Autodesk Inventor part; units mm, degrees
ref_plane "Work Plane4" through (164.3995, -80, 0) normal (0, 0, 1) x (1, 0, 0)
ref_plane "YZ Plane" through (0, 0, 0) normal (1, 0, 0) x (0, 1, 0)
ref_plane "XZ Plane" through (0, 0, 0) normal (0, 1, 0) x (-1, 0, 0)
ref_plane "Work Plane4" through (164.3995, -80, 0) normal (0, 0, 1) x (1, 0, 0)
sketch "Sketch1" plane through (164.3995, -80, 0) normal (0, 0, 1) x (1, 0, 0)
  circle A0 centre (-12.7, -38.1) radius 4.5
  circle A1 centre (-12.7, -12.7) radius 4.5
  circle A2 centre (-176.0991, -12.7) radius 4.5
  circle A3 centre (-176.0991, -38.1) radius 4.5
  line L0 (0, -50.8) -> (-188.7991, -50.8)
  line L1 (0, 0) -> (0, -50.8)
  line L2 (-188.7991, 0) -> (0, 0)
  line L3 (-188.7991, 0) -> (-188.7991, -50.8)
  circle A4 centre (-94.3995, 37) radius 4.7625
  circle A5 centre (-134.3995, 37) radius 2.489
  circle A6 centre (-54.3995, 37) radius 2.489
  line L4 (-26.3995, 25) -> (-162.3995, 25)
  line L5 (-26.3995, 49) -> (-26.3995, 25)
  line L6 (-162.3995, 49) -> (-26.3995, 49)
  line L7 (-162.3995, 25) -> (-162.3995, 49)
  line L8 (-26.3995, 25) -> (0, 0)
  line L9 (-162.3995, 25) -> (-188.7991, 0)
  point P0 (-94.3995, 0)
  dimension "d5" = 136
  dimension "d6" = 24
  dimension "d7" = 28
  dimension "d8" = 12
  dimension "d9" = 12
  dimension "d10" = 68
  dimension "d11" = 40
  dimension "d12" = 12
  dimension "d13" = 25
  dimension "d14" = 9.525
  dimension "d15" = 4.978
  dimension "d16" = 4.978
extrude "Extrusion1" add sketch "Sketch1" along normal blind 10
fillet "Fillet3" radius 2 8 edges at (70, -130.8, 10) (164.3995, -105.4, 10) (151.1998, -67.5, 10) (138, -43, 10) (70, -31, 10) (2, -43, 10) (-11.1998, -67.5, 10) (-24.3995, -105.4, 10)
properties part number "1136_RU Top Plate_V1" material "Aluminum"
Design review of the part built by this model. Coordinates are the model's own, in mm. A direction names the side the tool comes from. Coordinates: 2 decimals unless noted, no trailing zeros. Loops run counter-clockwise (first coordinate to the right, second up) from the corner with the lowest first, then second, coordinate; pieces in that order, holes last.
Q1. For pin 1 (3 mm diameter, centred on x = 30, y = -43, fed in from +Z); pin 2 (3 mm diameter, centred on y = -49, z = 6, fed in from +X), all flat-tipped, find the tip position at first contact; note any pin that passes through.
Reported:
pin 1: passes through
pin 2: stops at x = 138
Q2. To check wall thickness, follow line 1 (Y direction, x = 148.5, z = 5.75); line 2 (X direction, y = -121, z = 8.5); line 3 (Y direction, x = 110, z = 7). State the ranges of each line that lie inside material, in increasing order.
Reported:
line 1: y = -130.8 to -121.26, -114.94 to -95.86, -89.54 to -64.94
line 2: x = -24.34 to -15.14, -8.26 to 148.26, 155.14 to 164.34
line 3: y = -130.8 to -45.49, -40.51 to -31
Q3. The part is to be moulded in two halves that separate along Y. For faces 1 (the face through (-11.02, -67.33, 3.94)), 2 (the face through (155.992, -94.052, 4.93)), 3 (the face through (69, -80, 0)), 4 (the face through (-9.28, -96.494, 4.93)), say which applies: +Y half, -Y half, draft (parallel to the pull), parting line (faces both ways), or undercut.
Reported:
face 1: +Y half
face 2: undercut
face 3: draft
face 4: undercut
Q4. We need section D-D on y = -43. State the section outline as (x, z) points.
Reported:
outline: (2, 0) - (27.51, 0) - (27.51, 10) - (4, 10) arc R2 ccw to (2, 8) - close; (32.49, 0) - (65.24, 0) - (65.24, 10) - (32.49, 10) - close; (74.76, 0) - (107.51, 0) - (107.51, 10) - (74.76, 10) - close; (112.49, 0) - (138, 0) - (138, 8) arc R2 ccw to (136, 10) - (112.49, 10) - close
Q5. We need section A-A on y = -118.1. State the section outline as (x, z) points, and give its area (3 significant figures).
Reported:
outline: (-24.4, 0) - (-16.2, 0) - (-16.2, 10) - (-22.4, 10) arc R2 ccw to (-24.4, 8) - close; (-7.2, 0) - (147.2, 0) - (147.2, 10) - (-7.2, 10) - close; (156.2, 0) - (164.4, 0) - (164.4, 8) arc R2 ccw to (162.4, 10) - (156.2, 10) - close
area: 1,710 mm2
Q6. We need section B-B on z = 4.75. State the section outline as (x, y) points (1 decimal), and give its area (3 significant figures).
Reported:
outline: (-24.4, -130.8) - (164.4, -130.8) - (164.4, -80) - (138, -55) - (138, -31) - (2, -31) - (2, -55) - (-24.4, -80) - close; hole circle Ø9 at (-11.7, -118.1); hole circle Ø9 at (-11.7, -92.7); hole circle Ø5 at (30, -43); hole circle Ø9.5 at (70, -43); hole circle Ø5 at (110, -43); hole circle Ø9 at (151.7, -118.1); hole circle Ø9 at (151.7, -92.7)
area: 16,600 mm2
Q7. Tool access review of faces 5 (the face through (69, -31, 4)), 6 (the face through (138, -43, 4)): name each direction out of +Z, -Z, +X, -X, +Y, -Y from which nothing blocks a thin tool from reaching the whole face with its end or side.
Reported:
face 5: +Z, -Z, +X, -X, +Y
face 6: +Z, -Z, +X, +Y
Q8. We need section C-C on x = 30. State the section outline as (y, z) points.
Reported:
outline: (-130.8, 0) - (-45.49, 0) - (-45.49, 10) - (-128.8, 10) arc R2 ccw to (-130.8, 8) - close; (-40.51, 0) - (-31, 0) - (-31, 8) arc R2 ccw to (-33, 10) - (-40.51, 10) - close
